Input: part model. Units: mm. Frame: model coordinates. Face numbers are marked on the shaded views. A direction names the side the tool comes from. Give positions to 0.01 mm unless a question says otherwise; leave off trailing zeros. Loops run counter-clockwise (first coordinate to the right, second up) from the corner with the lowest first, then second, coordinate; pieces in that order, holes last. Notation, with made-up numbers: (80.5, 14) -> (103.5, 14) arc R27 cw to (103.5, 36) -> close; hole circle Ø9 at (80.5, 45.25). An arc over 180 degrees is marked (long way). Answer as a JSON object with one key per item and string values. Group by question number.
```python
from build123d import *

# Parameters (mm, degrees)
SKETCH_1_R          = 23.5
SKETCH_1_R_2        = 4.5
EXTRUDE_1_DEPTH     = 8
SKETCH_2_R          = 31
EXTRUDE_2_DEPTH     = 5
FILLET_1_R          = 0.5
SKETCH_3_R          = 27
CUT_EXTRUDE_1_DEPTH = 67.728373836


with BuildPart() as part:
    # 草图1 → 凸台-拉伸1 (new body)
    with BuildSketch(Plane(origin=(0, 0, 0), x_dir=(0, 0, -1), z_dir=(1, 0, 0))):
        with BuildLine():
            Line((42.2809162, 28.518838077), (42.2809162, -28.518838077))
            ThreePointArc((42.2809162, -28.518838077), (0, -51), (-42.2809162, -28.518838077))
            Line((-42.2809162, -28.518838077), (-42.2809162, 28.518838077))
            ThreePointArc((-42.2809162, 28.518838077), (0, 51), (42.2809162, 28.518838077))
        make_face()
        Circle(SKETCH_1_R, mode=Mode.SUBTRACT)
        with Locations((0, 41)):
            Circle(SKETCH_1_R_2, mode=Mode.SUBTRACT)
        with Locations((35.507041555, 20.5)):
            Circle(SKETCH_1_R_2, mode=Mode.SUBTRACT)
        with Locations((35.507041555, -20.5)):
            Circle(SKETCH_1_R_2, mode=Mode.SUBTRACT)
        with Locations((0, -41)):
            Circle(SKETCH_1_R_2, mode=Mode.SUBTRACT)
        with Locations((-35.507041555, -20.5)):
            Circle(SKETCH_1_R_2, mode=Mode.SUBTRACT)
        with Locations((-35.507041555, 20.5)):
            Circle(SKETCH_1_R_2, mode=Mode.SUBTRACT)
    extrude(amount=EXTRUDE_1_DEPTH)

    # 草图2 → 凸台-拉伸2 (add)
    with BuildSketch(Plane.ZY):
        with Locations(Location((0, 0, 0), (0, 0, 180))):
            Circle(SKETCH_2_R)
    extrude(amount=EXTRUDE_2_DEPTH)

    # 圆角1
    fillet_1_edges = [part.edges().sort_by_distance(p)[0] for p in [
        (-5, 0, 31),
    ]]
    fillet(fillet_1_edges, radius=FILLET_1_R)

    # 草图3 → 切除-拉伸1 (cut, through all)
    with BuildSketch(Plane(origin=(0, 0, 0), x_dir=(0, 0, -1), z_dir=(1, 0, 0))):
        Circle(SKETCH_3_R)
    extrude(amount=-CUT_EXTRUDE_1_DEPTH, mode=Mode.SUBTRACT)


solid = part.part
```
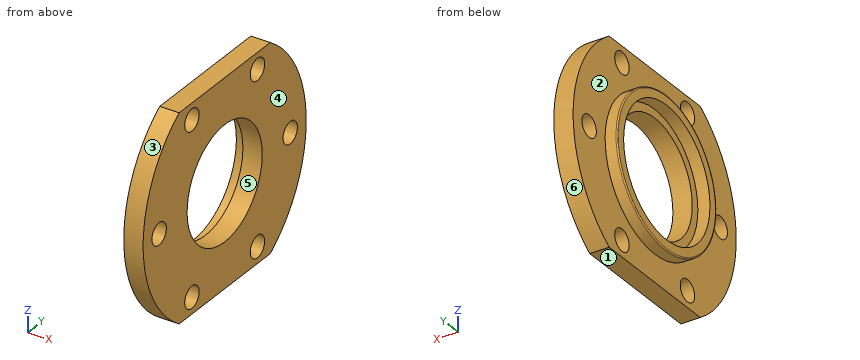
Q1. Section C-C on y = -43. Return the cut outline in (x, z), then the cut area to 3 significant figures.
Q2. Pull-direction query (Y, two-part tool) for the marked faces 3, 4, 5 and 6; classes: +Y half, -Y half, draft (parallel to the pull), parting line (faces both ways), or undercut.
Q3. Section B-B on z = -33. Return the cut outline in (x, y), then the cut area to 3 significant figures.
Q4. Set-up query: the marked faces 1 and 2. Return all of +Z, -Z, +X, -X, +Y, -Y with unobstructed straight access to the full face (end or side cutting, diameter ignored); none if empty.
Q5. Section A-A on x = 4.75. Return the cut outline in (y, z), then the cut area to 3 significant figures.
Q6. Ray query, probe 1 along Y at (x, z) = (0.5, 37.5); probe 2 along Z at (x, y) = (3.75, 21); probe 3 along Y at (x, z) = (-1.7, 0). Return the intervals inside material, ascending.
Q7. Pin query (flat end, axial travel): pin 1 Ø5 at (y, z) = (-12, -20.5) entering from -X; pin 2 Ø11.5 at (y, z) = (20.5, 35.51) entering from +X; pin 3 Ø2 at (x, z) = (1.5, -23.5) entering from -Y. Return the tip coordinate at first contact, or that it passes through.
Q8. Section D-D on y = 41. Return the cut outline in (x, z).
Numbers:
{
 "1": {"outline": "(0, -27.42) -> (8, -27.42) -> (8, -4.03) -> (0, -4.03) -> close; (0, 4.03) -> (8, 4.03) -> (8, 27.42) -> (0, 27.42) -> close", "area": "374 mm²"},
 "2": {"face 3": "-Y half", "face 4": "draft", "face 5": "undercut", "face 6": "+Y half"},
 "3": {"outline": "(0, -38.88) -> (8, -38.88) -> (8, -24.24) -> (0, -24.24) -> close; (0, -16.76) -> (8, -16.76) -> (8, 16.76) -> (0, 16.76) -> close; (0, 24.24) -> (8, 24.24) -> (8, 38.88) -> (0, 38.88) -> close", "area": "503 mm²"},
 "4": {"face 1": "-Z, +X, -X, +Y, -Y", "face 2": "-X"},
 "5": {"outline": "(-28.52, -42.28) -> (28.52, -42.28) arc R51 ccw to (28.52, 42.28) -> (-28.52, 42.28) arc R51 ccw to start; hole circle Ø9 at (-41, 0); hole circle Ø9 at (-20.5, -35.51); hole circle Ø9 at (-20.5, 35.51); hole circle Ø47 at (0, 0); hole circle Ø9 at (20.5, -35.51); hole circle Ø9 at (20.5, 35.51); hole circle Ø9 at (41, 0)", "area": "5,380 mm²"},
 "6": {"probe 1": "y = -34.57 to -24.53, -16.47 to 16.47, 24.53 to 34.57", "probe 2": "z = -42.28 to -39.98, -31.03 to -10.55, 10.55 to 31.03, 39.98 to 42.28", "probe 3": "y = -31 to -27, 27 to 31"},
 "7": {"pin 1": "stops at x = 0", "pin 2": "stops at x = 8", "pin 3": "stops at y = -45.77"},
 "8": {"outline": "(0, -30.33) -> (8, -30.33) -> (8, -4.5) -> (0, -4.5) -> close; (0, 4.5) -> (8, 4.5) -> (8, 30.33) -> (0, 30.33) -> close"}
}
